Geometry check sheet. Reference: the model listing, model coordinates, mm. A direction names the side the tool comes from. Coordinates: 2 decimals unless noted, no trailing zeros. Write each loop counter-clockwise with the first axis right and the second up, starting at its lowest first coordinate (ties: lowest second). Pieces come first, ordered by that corner, then holes. Notation, with made-up numbers: M -29,-37 L 5,-37 A20 cw 5,-21 Z; hole C 61.5,82.25 d7. An arc over 180 degrees is marked long. Put each result on its own line as item: value. Start each with the question number.
1) Gauge pin test, flat end, axial feed: pin 1 (3 mm diameter, centred on x = 34.5, z = 0.5, fed in from -Y). Record the tip position at first contact, or that the pin passes through.
2) Cross-section at A-A on z = 0. Record the cut outline in (x, y).
3) Cross-section at C-C on x = 12. Record the cut outline in (y, z), plus the area to 3 significant figures.
4) Scan lines: line 1 along X through (y, z) = (1.6, -0.1); line 2 along Z through (x, y) = (-22, -0.1); line 3 along Y through (x, z) = (-56, -2). Record each from-to range of solid material in increasing order.
5) Set-up check for faces 1 (the cylindrical face through (0.89, -2.44, 0.54)), 2 (the flat face through (-63.5, -2, 0)), 3 (the cylindrical face through (66.46, 0.07, 1.5)): record each of +Z, -Z, +X, -X, +Y, -Y from which the full face is reachable in a straight line by a thin tool's end or side.
from build123d import *

# Parameters (mm, degrees)
SKETCH1_R           = 2.5
BOSS_EXTRUDE1_DEPTH = 63.5
SKETCH2_R           = 1.5
BOSS_EXTRUDE2_DEPTH = 6
SKETCH3_R           = 1.5
BOSS_EXTRUDE3_DEPTH = 6


with BuildPart() as part:
    # Sketch1 → Boss-Extrude1 (new body, symmetric)
    with BuildSketch(Plane(origin=(0, 0, 0), x_dir=(0, 0, -1), z_dir=(1, 0, 0))):
        Circle(SKETCH1_R)
    extrude(amount=BOSS_EXTRUDE1_DEPTH, both=True)

    # Sketch2 → Boss-Extrude2 (add)
    with BuildSketch(Plane(origin=(63.5, 0, 0), x_dir=(0, 0, -1), z_dir=(1, 0, 0))):
        Circle(SKETCH2_R)
    extrude(amount=BOSS_EXTRUDE2_DEPTH)

    # Sketch3 → Boss-Extrude3 (add)
    with BuildSketch(Plane.ZY.offset(63.5)):
        Circle(SKETCH3_R)
    extrude(amount=BOSS_EXTRUDE3_DEPTH)


solid = part.part
Answer key:
1. pin 1: stops at y = -2.5
2. outline: M -69.5,-1.5 L -63.5,-1.5 L -63.5,-2.5 L 63.5,-2.5 L 63.5,-1.5 L 69.5,-1.5 L 69.5,1.5 L 63.5,1.5 L 63.5,2.5 L -63.5,2.5 L -63.5,1.5 L -69.5,1.5 Z
3. outline: C 0,0 d5
3. area: 19.6 mm²
4. line 1: x = -63.5 to 63.5
4. line 2: z = -2.5 to 2.5
4. line 3: y = -1.5 to 1.5
5. face 1: +X, -X
5. face 2: -X
5. face 3: +X
